Check sheet for the modelled part. Datum: model origin and axes. Units: mm. Face numbers are marked on the shaded views. A direction names the side the tool comes from. Round coordinates to 2 decimals unless told otherwise and drop trailing zeros. Order: outer loops, then holes, each group sorted by start corner. A loop starts at its lowest first (then second) coordinate and runs counter-clockwise, first axis right, second up.
Autodesk Inventor part; units mm, degrees
ref_plane "YZ Plane" through (0, 0, 0) normal (1, 0, 0) x (0, 1, 0)
ref_plane "XZ Plane" through (0, 0, 0) normal (0, 1, 0) x (-1, 0, 0)
ref_plane "XY Plane" through (0, 0, 0) normal (0, 0, 1) x (1, 0, 0)
sketch "草圖1" plane through (0, 0, 0) normal (0, 0, 1) x (1, 0, 0)
  circle A0 centre (0, 0) radius 12.85
  dimension "d0" = 25.7
extrude "擠出1" add sketch "草圖1" along normal blind 26
sketch "草圖2" plane through (0, 0, 26) normal (0, 0, 1) x (1, 0, 0)
  circle A0 centre (0, 0) radius 10
  circle A1 centre (0, 0) radius 12.85
  dimension "d3" = 20
extrude "擠出2" cut sketch "草圖2" against normal blind 1
sketch "草圖3" plane through (0, 0, 0) normal (0, 1, 0) x (-1, 0, 0)
  line L0 (-12.85, 25) -> (12.85, 25)
  line L1 (10, 26) -> (10, 25)
  line L2 (10, 25) -> (12.85, 21)
  line L3 (12.85, 0) -> (12.85, 25)
  line L4 (0, -5.2) -> (0, 31.2)
  point P0 (0, 0)
  dimension "d6" = 4
revolve "迴轉1" cut sketch "草圖3" angle 360 about axis through (0, 0, -10) along (0, 0, 1)
sketch "草圖4" plane through (0, 0, 0) normal (0, 0, -1) x (-1, 0, 0)
  circle A0 centre (0, 0) radius 5
  circle A1 centre (0, 0) radius 12.85
  dimension "d8" = 10
extrude "擠出3" cut sketch "草圖4" against normal blind 2
sketch "草圖5" plane through (0, 0, 2) normal (0, 0, -1) x (-1, 0, 0)
  circle A0 centre (0, 0) radius 10.5
  circle A1 centre (0, 0) radius 12.85
  dimension "d11" = 21
extrude "擠出4" cut sketch "草圖5" against normal blind 3
sketch "草圖6" plane through (0, 0, 2) normal (0, 0, -1) x (-1, 0, 0)
  line L0 (0, 0) -> (-13.3502, 0) construction
  line L1 (0, 0) -> (8.2303, -14.2554) construction
  line L2 (0, 0) -> (8.5219, 14.7603) construction
  line L3 (-10.3078, -2) -> (-4.5826, -2)
  line L4 (-10.3078, 2) -> (-4.5826, 2)
  circle A0 centre (0, 0) radius 5
  circle A1 centre (0, 0) radius 10.5
  line L5 (0.5592, -4.9686) -> (3.4218, -9.9268)
  line L6 (4.0233, -2.9686) -> (6.8859, -7.9268)
  line L7 (4.0233, 2.9686) -> (6.8859, 7.9268)
  line L8 (0.5592, 4.9686) -> (3.4218, 9.9268)
  dimension "d14" = 120
  dimension "d15" = 120
  dimension "d16" = 2
  dimension "d17" = 2
  dimension "d18" = 4
  dimension "d19" = 2
  dimension "d20" = 2
  dimension "d21" = 2
extrude "擠出5" cut sketch "草圖6" against normal blind 10 contours L3 A0 L5 A1 | A1 L8 A0 L4 | L6 A0 L7 A1
fillet "圓角1" radius 3 3 edges at (10.5, 0, 2) (-5.25, 9.0933, 2) (-5.25, -9.0933, 2)
sketch "草圖8" plane through (0, 0, 0) normal (0, 1, 0) x (-1, 0, 0)
  line L0 (-12.85, 5) -> (-12.85, 5.6297)
  line L1 (0, -5.2) -> (0, 31.2)
  line L2 (-12.85, 5.6297) -> (-10.5, 5)
  line L3 (12.85, 5) -> (-12.85, 5)
  line L4 (-10.5, 5) -> (-10.3078, 5)
  point P0 (0, 0)
  dimension "d28" = 15
revolve "迴轉2" cut sketch "草圖8" angle 360 about axis through (0, 0, -10) along (0, 0, 1)
sketch "草圖9" plane through (0, 0, 26) normal (0, 0, 1) x (1, 0, 0)
  circle A0 centre (0, 0) radius 9.5
  dimension "d29" = 19
extrude "擠出6" add sketch "草圖9" along normal blind 21.787
equation "\"d15\" = d14"
equation "\"d17\" = d16"
equation "\"d20\" = d19"
equation "\"d21\" = d19"
properties part number "moter"
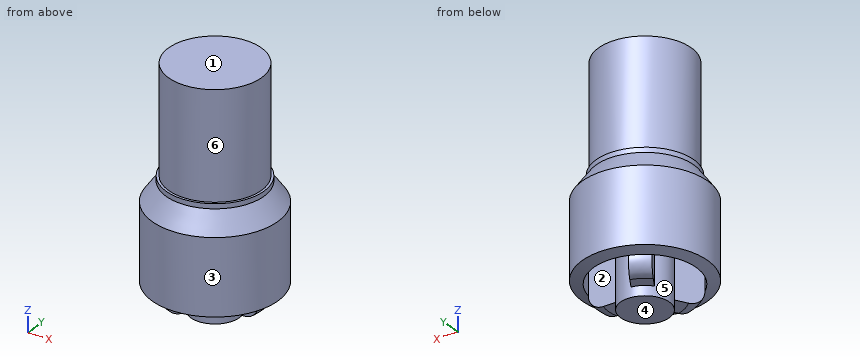
Item 1: Sectioned sample at C-C (z = 10.5). Record the cut outline in (x, y).
Answer:
outline: circle Ø25.7 at (0, 0); hole (-6.89, -7.93) - (-4.02, -2.97) arc R5 cw to (-4.02, 2.97) - (-6.89, 7.93) arc R10.5 ccw to start; hole (-3.42, -9.93) arc R10.5 ccw to (10.31, -2) - (4.58, -2) arc R5 cw to (-0.56, -4.97) - close; hole (-3.42, 9.93) - (-0.56, 4.97) arc R5 cw to (4.58, 2) - (10.31, 2) arc R10.5 ccw to start
Item 2: Scan lines: line 1 along Y through (x, z) = (6.5, 11.5); line 2 along X through (y, z) = (-5.25, 10); line 3 along Z through (x, y) = (4, 7.5). Record each from-to range of solid material in increasing order.
Answer:
line 1: y = -11.08 to -8.25, -2 to 2, 8.25 to 11.08
line 2: x = -11.73 to -9.09, -5.34 to -0.72, 9.09 to 11.73
line 3: z = 12 to 47.79
Item 3: Go/stop test with flat-tipped pins: P1, Ø1, axis at x = -1.5, y = 7, coming from the -Z side; P2, Ø1.9, axis at x = -6.5, y = 2.5, coming from the -Z side; P3, Ø4, axis at x = -4.5, z = 21.5, coming from the -Y side. Record where each tip stops, or that it passes through.
Answer:
P1: stops at z = 2
P2: stops at z = 12
P3: stops at y = -12.59
Item 4: Sectioned sample at D-D (z = 40). Record the cut outline in (x, y), and give its area (3 significant figures).
Answer:
outline: circle Ø19 at (0, 0)
area: 284 mm2
Item 5: Access from +Z, -Z, +X, -X, +Y, -Y to the whole of each face (thin tool, end or side, straight path). Record for the marked faces 4, 5 and 6.
Answer:
face 4: -Z, +X, -X, +Y, -Y
face 5: -Z
face 6: +Z
Item 6: Release check for a two-part mould opening along Y. For the marked faces 1, 2 and 3 record: released by +Y, released by -Y, zero draft, split by the parting line, or undercut.
Answer:
face 1: zero draft
face 2: undercut
face 3: split by the parting line
Item 7: Sectioned sample at A-A (x = 0). Record the cut outline in (y, z).
Answer:
outline: (-12.85, 5.63) - (-10.5, 5) - (-10.5, 12) - (-5, 12) - (-5, 0) - (5, 0) - (5, 12) - (10.5, 12) - (10.5, 5) - (12.85, 5.63) - (12.85, 21) - (10, 25) - (10, 26) - (9.5, 26) - (9.5, 47.79) - (-9.5, 47.79) - (-9.5, 26) - (-10, 26) - (-10, 25) - (-12.85, 21) - close
